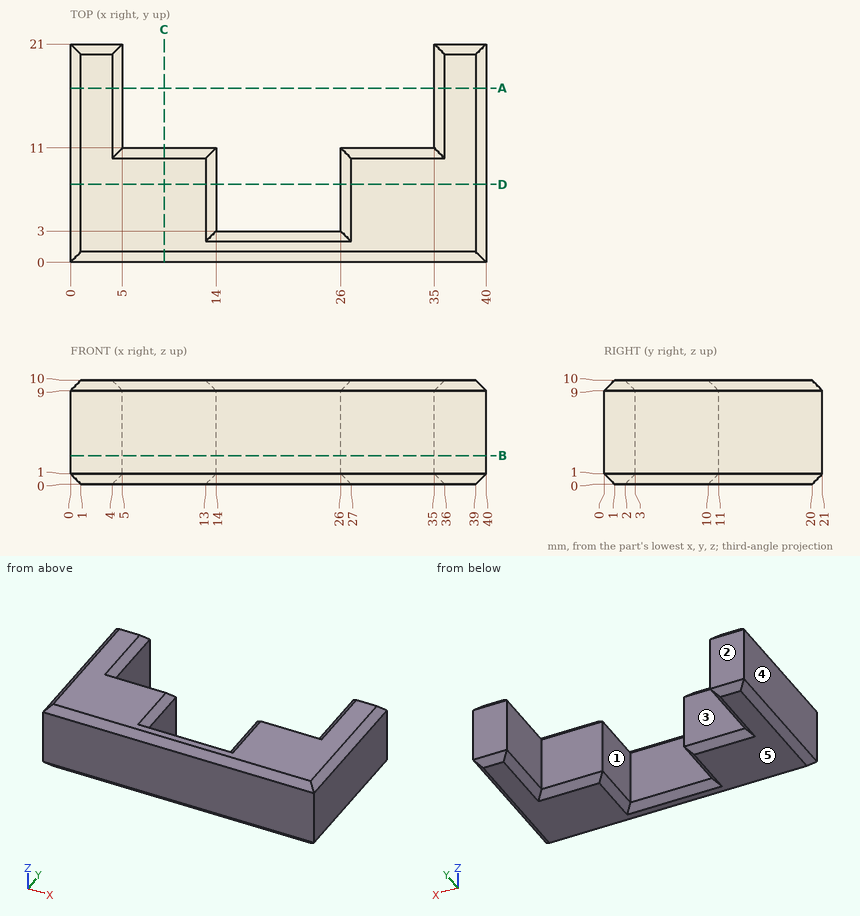
Can you work these out from the drawing? Everything is in mm from the part's minimum corner. A direction names the side the tool comes from. Round coordinates to 2 decimals unless told otherwise and drop trailing zeros. Order: outer loops, then holes, each group sorted by start corner. A loop starts at its lowest first (then second) coordinate and runs counter-clockwise, first axis right, second up. Notation, with made-up numbers: (48.5, -23) -> (78.5, -23) arc R8 cw to (78.5, -16) -> close; hole circle Ø6 at (64, 36.25). An arc over 180 degrees is marked (long way). Use CSV: the item, a comma, the result in double quotes.
1. Which directions (+Z, -Z, +X, -X, +Y, -Y) give clear straight access to the entire face, cutting with the end or side of a thin tool? Please do the marked faces 1 and 2.
Recorded:
face 1,"+Z, -Z, +Y"
face 2,"+Z, -Z, +X, -X, +Y"
2. I want a section at C-C on x = 9. List the corners of the cut face in (y, z) for me, and give its area (3 significant figures).
Recorded:
outline,"(0, 1) -> (1, 0) -> (10, 0) -> (11, 1) -> (11, 9) -> (10, 10) -> (1, 10) -> (0, 9) -> close"
area,"108 mm2"
3. I want a section at B-B on z = 2.75. List the corners of the cut face in (x, y) for me, and give its area (3 significant figures).
Recorded:
outline,"(0, 0) -> (40, 0) -> (40, 21) -> (35, 21) -> (35, 11) -> (26, 11) -> (26, 3) -> (14, 3) -> (14, 11) -> (5, 11) -> (5, 21) -> (0, 21) -> close"
area,"444 mm2"
4. I want a section at D-D on y = 7.5. List the corners of the cut face in (x, z) for me, and give its area (3 significant figures).
Recorded:
outline,"(0, 1) -> (1, 0) -> (13, 0) -> (14, 1) -> (14, 9) -> (13, 10) -> (1, 10) -> (0, 9) -> close; (26, 1) -> (27, 0) -> (39, 0) -> (40, 1) -> (40, 9) -> (39, 10) -> (27, 10) -> (26, 9) -> close"
area,"276 mm2"
5. Thinking about a two-plate mould opening in X: for the marked faces 3, 4 and 5, which applies, pulls with the +X half, pulls with the -X half, needs draft (parallel to the pull), parting line crosses it, or undercut?
Recorded:
face 3,"undercut"
face 4,"pulls with the -X half"
face 5,"needs draft"
6. I'm going to push flat-ended pins straight in: P1, Ø4, axis at x = 11.5, z = 5, coming from the +Y side; P2, Ø2, axis at x = 16, z = 2.5, coming from the +Y side. Where does each tip first touch, or does it pass through?
Recorded:
P1,"stops at y = 11"
P2,"stops at y = 3"
7. I need wall thicknesses on line 1 along X through (y, z) = (17, 7); line 2 along X through (y, z) = (7.75, 1.5); line 3 along Y through (x, z) = (24.5, 3). Which ranges of each line are inside material? Lowest first, please.
Recorded:
line 1,"x = 0 to 5, 35 to 40"
line 2,"x = 0 to 14, 26 to 40"
line 3,"y = 0 to 3"
8. I want a section at A-A on y = 16.75. List the corners of the cut face in (x, z) for me.
Recorded:
outline,"(0, 1) -> (1, 0) -> (4, 0) -> (5, 1) -> (5, 9) -> (4, 10) -> (1, 10) -> (0, 9) -> close; (35, 1) -> (36, 0) -> (39, 0) -> (40, 1) -> (40, 9) -> (39, 10) -> (36, 10) -> (35, 9) -> close"
